Check sheet for the modelled part. Datum: model origin and axes. Units: mm. A direction names the side the tool comes from. Coordinates: 2 decimals unless noted, no trailing zeros. Loops run counter-clockwise (first coordinate to the right, second up) from the corner with the lowest first, then second, coordinate; pieces in that order, holes last.
from build123d import *

# Parameters (mm, degrees)
F2_W          = 10
F2_H          = 10
F3_DEPTH      = 100
F3_DEPTH_BACK = 100
F4_W          = 10
F4_H          = 10
F5_DEPTH      = 50
F5_DEPTH_BACK = 50


with BuildPart() as f1:
    # F0 (on Front) → F1 (revolve)
    with BuildSketch(Plane.XZ):
        Polygon((0, 29), (0, 20), (4, 20), (4, 21.5), (14, 21.5), (14, 20), (38, 20), (38, 22), (31, 24), (16, 24), (16, 29), (14, 29), (14, 26.5), (4, 26.5), (4, 29), align=None)
    revolve(axis=Axis((36.8667048862, 0, 0), (1, 0, 0)))

    # F2 (on Front) → F3 (cut, two sides)
    with BuildSketch(Plane.XZ) as f3_sk:
        with Locations((9, 0)):
            Rectangle(F2_W, F2_H)
    extrude(amount=-F3_DEPTH, mode=Mode.SUBTRACT)
    extrude(f3_sk.sketch, amount=F3_DEPTH_BACK, mode=Mode.SUBTRACT)

    # F4 (on Top) → F5 (cut, two sides)
    with BuildSketch(Plane.XY) as f5_sk:
        with Locations((9, 0)):
            Rectangle(F4_W, F4_H)
    extrude(amount=-F5_DEPTH, mode=Mode.SUBTRACT)
    extrude(f5_sk.sketch, amount=F5_DEPTH_BACK, mode=Mode.SUBTRACT)


solid = f1.part
(1) Section check A-A, the plane z = 0. Enter the section's corners in (x, y).
(2) Scan lines: line 1 along Y through (x, z) = (30, 0); line 2 along Y through (x, z) = (2, 0). Record each from-to range of solid material in increasing order.
(3) Draft check along X on faces 4 (the face through (37.562, -6.646, 21.103)), 5 (the face through (9, 23, -5)), 6 (the face through (8.93, -18.894, -18.581)), 7 (the face through (26.168, 19.524, -4.336)). Enter one of: pulls with the +X half, pulls with the -X half, needs draft (parallel to the pull), parting line crosses it, or undercut.
(4) Set-up check for faces 1 (the face through (9.07, -15.085, 15.32)), 2 (the face through (9, 5, 23)), 3 (the face through (8.93, -18.581, 18.894)): record each of +Z, -Z, +X, -X, +Y, -Y from which the full face is reachable in a straight line by a thin tool's end or side.
(5) Gauge pin test, flat ends, axial feed: P1, Ø5, axis at x = 23, z = 15, coming from the -Y side; P2, Ø4, axis at x = 7.5, y = -24.5, coming from the +Z side; P3, Ø5.5, axis at x = 11, z = 23, coming from the -Y side; P4, Ø17.5, axis at y = 5.5, z = -6, coming from the +X side. Record the tip position at first contact, or that the pin passes through.
(6) Section check D-D, the plane y = 25. Enter the section's corners in (x, z), plus the area to 3 significant figures.
(7) Section check B-B, the plane x = 7.5. Enter the section's corners in (y, z), plus the area to 3 significant figures.
Determined:
1. outline: (0, -29) - (4, -29) - (4, -20) - (0, -20) - close; (0, 20) - (4, 20) - (4, 29) - (0, 29) - close; (14, -29) - (16, -29) - (16, -24) - (31, -24) - (38, -22) - (38, -20) - (14, -20) - close; (14, 20) - (38, 20) - (38, 22) - (31, 24) - (16, 24) - (16, 29) - (14, 29) - close
2. line 1: y = -24 to -20, 20 to 24
2. line 2: y = -29 to -20, 20 to 29
3. face 4: pulls with the +X half
3. face 5: undercut
3. face 6: undercut
3. face 7: needs draft
4. face 1: none
4. face 2: +Z, -Z
4. face 3: +Z, -Y
5. P1: stops at y = -20.49
5. P2: stops at z = 14
5. P3: stops at y = -17.09
5. P4: passes through
6. outline: (0, -14.7) - (4, -14.7) - (4, -8.79) - (14, -8.79) - (14, -14.7) - (16, -14.7) - (16, 14.7) - (14, 14.7) - (14, 8.79) - (4, 8.79) - (4, 14.7) - (0, 14.7) - close; hole (4, -5) - (14, -5) - (14, 5) - (4, 5) - close
6. area: 252 mm2
7. outline: (-26.02, -5) arc R26.5 ccw to (-5, -26.02) - (-5, -20.91) arc R21.5 cw to (-20.91, -5) - close; (-26.02, 5) - (-20.91, 5) arc R21.5 cw to (-5, 20.91) - (-5, 26.02) arc R26.5 ccw to start; (5, -26.02) arc R26.5 ccw to (26.02, -5) - (20.91, -5) arc R21.5 cw to (5, -20.91) - close; (5, 20.91) arc R21.5 cw to (20.91, 5) - (26.02, 5) arc R26.5 ccw to (5, 26.02) - close
7. area: 552 mm2
